Build history of the part. All positions in model axes, mm. A direction names the side the tool comes from. Coordinates: 2 decimals unless noted, no trailing zeros. Write each loop counter-clockwise with the first axis right and the second up, starting at its lowest first coordinate (ties: lowest second). Pieces come first, ordered by that corner, then holes.
from build123d import *

# Parameters (mm, degrees)
F0_W     = 25.4
F0_H     = 25.4
F1_DEPTH = 12.7
F2_R     = 8.3183998394
F3_DEPTH = 25.4
F4_R     = 5.08
F6_D     = 2.2606
F6_DEPTH = 14.605
F6_TIP   = 0.6791527577


with BuildPart() as f1:
    # F0 (on Front) → F1 (new body)
    with BuildSketch(Plane.XZ):
        Rectangle(F0_W, F0_H)
    extrude(amount=F1_DEPTH)

    # F2 (on face) → F3 (join)
    with BuildSketch(Plane.XZ.offset(12.7)):
        Circle(F2_R)
    extrude(amount=F3_DEPTH)

    # F4
    f4_edges = [f1.edges().sort_by_distance(p)[0] for p in [
        (-12.7, -6.35, -12.7),
    ]]
    fillet(f4_edges, radius=F4_R)

    # F6
    with Locations(Plane(origin=(0, 0, 0), x_dir=(-1, 0, 0), z_dir=(0, 1, 0))):
        with Locations((0, 0)):
            Hole(F6_D / 2, depth=F6_DEPTH)
            with Locations((0, 0, -(F6_DEPTH + F6_TIP / 2))):  # 118° drill point
                Cone(0, F6_D / 2, F6_TIP, mode=Mode.SUBTRACT)


solid = f1.part
(1) Slice it at C-C, the plane y = -29. List the corners of the cut face in (x, z), and give its area (3 significant figures).
(2) Two-plate mould, pull along Z, no slides. Class faces 3 (the flat face through (-12.7, -6, 2)), 4 (the cylindrical face through (-0.245, -7.405, -1.103)), 5 (the cylindrical face through (-11.251, -6.439, -11.172)): pulls with the +Z half, pulls with the -Z half, needs draft (parallel to the pull), parting line crosses it, or undercut.
(3) Flat gauge pins, fed straight in: P1, Ø1.5, axis at y = -15, z = -6.5, coming from the -X side; P2, Ø12, axis at y = -28.5, z = 4.5, coming from the +X side; P3, Ø8, axis at x = 9, y = -21.5, coming from the -Z side. Where does each tip first touch, or does it go through?
(4) Slice it at D-D, the plane x = 11.25. List the corners of the cut face in (y, z), and give its area (3 significant figures).
(5) 3-axis set-ups, long thin cutter, end or side, ignore diameter. For faces 1 (the flat face through (0, -12.7, 9)), 2 (the conical face through (0.156, -15.166, -0.119)): which of +Z, -Z, +X, -X, +Y, -Y reach the whole face in a straight line?
(6) Slice it at B-B, the plane x = -3.75. List the corners of the cut face in (y, z).
(7) Probe L1, parallel to X at y = -3.5, z = 0; L2, parallel to Y at x = -11, z = 10.5. List the from-to ranges inside material, lowest first.
(8) Slice it at A-A, the plane z = 2.5. List the corners of the cut face in (x, y).
Results:
1. outline: circle Ø16.64 at (0, 0)
1. area: 217 mm2
2. face 3: needs draft
2. face 4: undercut
2. face 5: pulls with the -Z half
3. P1: stops at x = -6.01
3. P2: stops at x = 8.32
3. P3: stops at z = -6.65
4. outline: (-12.7, -12.7) - (0, -12.7) - (0, 12.7) - (-12.7, 12.7) - close
4. area: 323 mm2
5. face 1: -Y
5. face 2: +Y
6. outline: (-38.1, -7.43) - (-12.7, -7.43) - (-12.7, -12.7) - (0, -12.7) - (0, 12.7) - (-12.7, 12.7) - (-12.7, 7.43) - (-38.1, 7.43) - close
7. L1: x = -12.7 to -1.13, 1.13 to 12.7
7. L2: y = -12.7 to 0
8. outline: (-12.7, -12.7) - (-7.93, -12.7) - (-7.93, -38.1) - (7.93, -38.1) - (7.93, -12.7) - (12.7, -12.7) - (12.7, 0) - (-12.7, 0) - close
